Geometry: final body of the model. Coordinates: model frame, mm. A direction names the side the tool comes from. Give positions to 0.01 mm unless a question says otherwise; leave off trailing zeros. Order: outer loops, then holes, each group sorted by start corner. A loop starts at its lowest first (then second) coordinate and runs counter-clockwise, first axis right, second up. Notation, with made-up numbers: (-21, 20.25) -> (2, 20.25) arc R20 ccw to (2, 34.25) -> close; hole circle Ø11 at (-27, 62). An arc over 180 degrees is marked (long way). One line per question, with ' | ' between items. Start each with the question number.
(1) Mould query, pull axis X, two halves, no side actions, for faces 1 (the face through (-13.695, 59, 18)), 2 (the face through (13.38, 7.57, 13.29)), 3 (the face through (-15.5, 6.2, 0)). Classes: +X half, -X half, draft (parallel to the pull), parting line (faces both ways), or undercut.
(2) Section B-B (x = 0). Return loops of the section in (y, z) (3 decimals), then the cut area to 3 significant figures.
(3) Section A-A (z = 20). Return loops of the section in (x, y).
(4) Section D-D (x = 25). Return loops of the section in (y, z).
(5) First-contact query: pin 1 Ø4 at (y, z) = (-71.5, 20) entering from -X; pin 2 Ø8 at (x, z) = (10, 17.5) entering from -Y; pin 3 Ø4 at (y, z) = (66.5, 18) entering from +X; pin 4 Ø16 at (x, y) = (0, 0) entering from -Z. Flat tips, straight axial feed; report the tip coordinate or a pass-through.
(6) Ray query, L1, parallel to Y at x = -0.5, z = 1.75 (3 decimals); L2, parallel to Z at x = 2.5, y = 74.5; L3, parallel to Y at x = 0, z = 18.5. Return the intervals inside material, ascending.
(7) Section C-C (y = 78.5). Return loops of the section in (x, z), then the cut area to 3 significant figures.
(8) Set-up query: faces 4 (the face through (-13.248, 7.799, 13.287)), 5 (the face through (-13.695, -58, 18)), 6 (the face through (13.695, 58, 18)). Return all of +Z, -Z, +X, -X, +Y, -Y with unobstructed straight access to the full face (end or side cutting, diameter ignored); none if empty.
```python
from build123d import *

# Parameters (mm, degrees)
F0_R     = 20.75
F1_DEPTH = 14
F3_DEPTH = 8
F4_R     = 13.133574
F5_DEPTH = 25
F6_R     = 2.5


with BuildPart() as f1:
    # F0 (on Top) → F1 (new body)
    with BuildSketch(Plane.XY):
        Circle(F0_R)
        Polygon((-18.619546, 0), (-9.309773, 16.125), (9.309773, 16.125), (18.619546, 0), (9.309773, -16.125), (-9.309773, -16.125), align=None, mode=Mode.SUBTRACT)
    extrude(amount=F1_DEPTH)

    # F2 (on face) → F3 (join)
    with BuildSketch(Plane.XY.offset(14)):
        with BuildLine():
            Line((-13.69534, 91.853356), (-13.69534, 25.562427))
            ThreePointArc((-13.69534, 25.562427), (-29, 0), (-13.69534, -25.562427))
            Line((-13.69534, -25.562427), (-13.69534, -91.853356))
            ThreePointArc((-13.69534, -91.853356), (-10.766407, -98.924424), (-3.69534, -101.853356))
            Line((-3.69534, -101.853356), (3.69534, -101.853356))
            ThreePointArc((3.69534, -101.853356), (10.766407, -98.924424), (13.69534, -91.853356))
            Line((13.69534, -91.853356), (13.69534, -25.562427))
            ThreePointArc((13.69534, -25.562427), (29, 0), (13.69534, 25.562427))
            Line((13.69534, 25.562427), (13.69534, 91.853356))
            ThreePointArc((13.69534, 91.853356), (10.766407, 98.924424), (3.69534, 101.853356))
            Line((3.69534, 101.853356), (-3.69534, 101.853356))
            ThreePointArc((-3.69534, 101.853356), (-10.766407, 98.924424), (-13.69534, 91.853356))
        make_face()
    extrude(amount=F3_DEPTH)

    # F4 (on face) → F5 (cut)
    with BuildSketch(Plane.XY.offset(22)):
        Circle(F4_R)
    extrude(amount=-F5_DEPTH, mode=Mode.SUBTRACT)

    # F6
    f6_edges = [f1.edges().sort_by_distance(p)[0] for p in [
        (0, 16.125, 14),
        (-13.96466, 8.0625, 14),
        (-13.96466, -8.0625, 14),
        (0, -16.125, 14),
        (13.96466, -8.0625, 14),
        (13.96466, 8.0625, 14),
        (-20.75, 0, 14),
    ]]
    fillet(f6_edges, radius=F6_R)


solid = f1.part
```
Response:
1) face 1: -X half | face 2: undercut | face 3: draft
2) outline: (-101.853, 14) -> (-23.25, 14) arc R2.5 cw to (-20.75, 11.5) -> (-20.75, 0) -> (-16.125, 0) -> (-16.125, 11.5) arc R2.5 cw to (-13.625, 14) -> (-13.134, 14) -> (-13.134, 22) -> (-101.853, 22) -> close; (13.134, 14) -> (13.625, 14) arc R2.5 cw to (16.125, 11.5) -> (16.125, 0) -> (20.75, 0) -> (20.75, 11.5) arc R2.5 cw to (23.25, 14) -> (101.853, 14) -> (101.853, 22) -> (13.134, 22) -> close | area: 1,550 mm^2
3) outline: (-13.7, -91.85) arc R10 ccw to (-3.7, -101.85) -> (3.7, -101.85) arc R10 ccw to (13.7, -91.85) -> (13.7, -25.56) arc R29 ccw to (13.7, 25.56) -> (13.7, 91.85) arc R10 ccw to (3.7, 101.85) -> (-3.7, 101.85) arc R10 ccw to (-13.7, 91.85) -> (-13.7, 25.56) arc R29 ccw to (-13.7, -25.56) -> close; hole circle Ø26.27 at (0, 0)
4) outline: (-14.7, 14) -> (14.7, 14) -> (14.7, 22) -> (-14.7, 22) -> close
5) pin 1: stops at x = -13.7 | pin 2: stops at y = -101.58 | pin 3: stops at x = 13.7 | pin 4: passes through
6) L1: y = -20.744 to -16.125, 16.125 to 20.744 | L2: z = 14 to 22 | L3: y = -101.85 to -13.13, 13.13 to 101.85
7) outline: (-13.7, 14) -> (13.7, 14) -> (13.7, 22) -> (-13.7, 22) -> close | area: 219 mm^2
8) face 4: -Z | face 5: +Z, -Z, -X, -Y | face 6: +Z, -Z, +X, +Y
